```python
from build123d import *

# Parameters (mm, degrees)
SKETCH1_R           = 1.6
BOSS_EXTRUDE1_DEPTH = 3.175
SKETCH2_R           = 1.6
SKETCH2_R_2         = 7.5
CUT_EXTRUDE1_DEPTH  = 4.175


with BuildPart() as part:
    # Sketch1 → Boss-Extrude1 (new body)
    with BuildSketch(Plane.XY):
        with BuildLine():
            Line((31.086717458, 32.79124845), (24.539210672, 37.049362302))
            ThreePointArc((24.539210672, 37.049362302), (22.268882249, 37.695107847), (20.029743315, 36.948358029))
            Line((20.029743315, 36.948358029), (13.602836128, 32.346493758))
            ThreePointArc((13.602836128, 32.346493758), (12.968237383, 31.781029757), (12.467444066, 31.094246563))
            Line((12.467444066, 31.094246563), (1.349560594, 11.837507517))
            ThreePointArc((1.349560594, 11.837507517), (0.995156132, 11.028730142), (0.826837821, 10.16190126))
            Line((0.826837821, 10.16190126), (0.217529035, 2.673448792))
            ThreePointArc((0.217529035, 2.673448792), (0.712425098, 0.398045931), (2.390731369, -1.216162343))
            Line((2.390731369, -1.216162343), (9.39530455, -4.779380795))
            ThreePointArc((9.39530455, -4.779380795), (10.276421795, -5.10394936), (11.208926603, -5.214163404))
            Line((11.208926603, -5.214163404), (33.291073397, -5.214163404))
            ThreePointArc((33.291073397, -5.214163404), (34.223578205, -5.10394936), (35.10469545, -4.779380795))
            Line((35.10469545, -4.779380795), (42.181392008, -1.179473262))
            ThreePointArc((42.181392008, -1.179473262), (43.83187157, 0.385744129), (44.362149812, 2.597710054))
            Line((44.362149812, 2.597710054), (43.941412908, 10.526262814))
            ThreePointArc((43.941412908, 10.526262814), (43.781938908, 11.451617014), (43.411134666, 12.314296889))
            Line((43.411134666, 12.314296889), (32.370061269, 31.437996983))
            ThreePointArc((32.370061269, 31.437996983), (31.808360702, 32.190462814), (31.086717458, 32.79124845))
        make_face()
        with Locations((13.589745962, 17.846043489)):
            Circle(SKETCH1_R, mode=Mode.SUBTRACT)
        with Locations((9.526279442, 5.5)):
            Circle(SKETCH1_R, mode=Mode.SUBTRACT)
        with Locations((34.973720558, 5.5)):
            Circle(SKETCH1_R, mode=Mode.SUBTRACT)
        with Locations((30.910254038, 17.846043489)):
            Circle(SKETCH1_R, mode=Mode.SUBTRACT)
        with Locations((22.25, 27.538130468)):
            Circle(SKETCH1_R, mode=Mode.SUBTRACT)
        with Locations((22.25, 2.846043489)):
            Circle(SKETCH1_R, mode=Mode.SUBTRACT)
        with BuildLine():
            Line((42.370834875, 9.312177826), (35.370834875, -2.812177826))
            ThreePointArc((35.370834875, -2.812177826), (34.687822174, -2.995190528), (34.504809472, -2.312177826))
            Line((34.504809472, -2.312177826), (41.504809472, 9.812177826))
            ThreePointArc((41.504809472, 9.812177826), (42.187822174, 9.995190528), (42.370834875, 9.312177826))
        make_face(mode=Mode.SUBTRACT)
        with BuildLine():
            Line((10.01754221, -2.349929674), (3.01754221, 9.774425979))
            ThreePointArc((3.01754221, 9.774425979), (2.334529508, 9.957438681), (2.151516806, 9.274425979))
            Line((2.151516806, 9.274425979), (9.151516806, -2.849929674))
            ThreePointArc((9.151516806, -2.849929674), (9.834529508, -3.032942376), (10.01754221, -2.349929674))
        make_face(mode=Mode.SUBTRACT)
        with BuildLine():
            Line((15.358452868, 31.038130468), (29.358452868, 31.038130468))
            ThreePointArc((29.358452868, 31.038130468), (29.858452868, 31.538130468), (29.358452868, 32.038130468))
            Line((29.358452868, 32.038130468), (15.358452868, 32.038130468))
            ThreePointArc((15.358452868, 32.038130468), (14.858452868, 31.538130468), (15.358452868, 31.038130468))
        make_face(mode=Mode.SUBTRACT)
    extrude(amount=BOSS_EXTRUDE1_DEPTH)

    # Sketch2 → Cut-Extrude1 (cut, through all)
    with BuildSketch(Plane.XY.offset(3.175)):
        with Locations((41.761034996, 1.563830145)):
            Circle(SKETCH2_R)
        with Locations((2.789891826, 1.563830145)):
            Circle(SKETCH2_R)
        with Locations((22.275463411, 12.813830145)):
            Circle(SKETCH2_R_2)
        with Locations((22.275463411, 35.313830145)):
            Circle(SKETCH2_R)
    extrude(amount=-CUT_EXTRUDE1_DEPTH, mode=Mode.SUBTRACT)


solid = part.part
```
Geometry check sheet. Reference: the model listing, model coordinates, mm. A direction names the side the tool comes from. Coordinates: 2 decimals unless noted, no trailing zeros. Order: outer loops, then holes, each group sorted by start corner. A loop starts at its lowest first (then second) coordinate and runs counter-clockwise, first axis right, second up. Notation, with made-up numbers: (-29, -33.5) - (-24, -33.5) arc R20 ccw to (-24, -14.5) - close; hole circle Ø10 at (81, 64). An arc over 180 degrees is marked (long way). Use one line per item in the form item = value.
1. Draft check along X on faces 3 (the face through (10.26, -5.1, 1.57)), 4 (the face through (42.18, 10, 1.57)), 5 (the face through (43.786, 11.439, 1.565)). Enter one of: pulls with the +X half, pulls with the -X half, needs draft (parallel to the pull), parting line crosses it, or undercut.
Here are the results:
face_3 = pulls with the -X half
face_4 = undercut
face_5 = pulls with the +X half
2. Section check B-B (y = 14). Record the boundary of the cut face in (x, z) (3 decimals).
Here are the results:
outline = (2.598, 0) - (14.87, 0) - (14.87, 3.175) - (2.598, 3.175) - close; (29.681, 0) - (42.438, 0) - (42.438, 3.175) - (29.681, 3.175) - close
3. Section check D-D (x = 38). Record the boundary of the cut face in (y, z) (3 decimals), then the cut area to 3 significant figures.
Here are the results:
outline = (-3.307, 0) - (1.742, 0) - (1.742, 3.175) - (-3.307, 3.175) - close; (3.742, 0) - (21.687, 0) - (21.687, 3.175) - (3.742, 3.175) - close
area = 73.0 mm²
4. Section check C-C (x = 23). Record the boundary of the cut face in (y, z) (3 decimals), then the cut area to 3 significant figures.
Here are the results:
outline = (-5.214, 0) - (1.433, 0) - (1.433, 3.175) - (-5.214, 3.175) - close; (4.259, 0) - (5.349, 0) - (5.349, 3.175) - (4.259, 3.175) - close; (20.279, 0) - (26.125, 0) - (26.125, 3.175) - (20.279, 3.175) - close; (28.951, 0) - (31.038, 0) - (31.038, 3.175) - (28.951, 3.175) - close; (32.038, 0) - (33.887, 0) - (33.887, 3.175) - (32.038, 3.175) - close; (36.74, 0) - (37.644, 0) - (37.644, 3.175) - (36.74, 3.175) - close
area = 58.5 mm²
5. Scan lines: line 1 (Y direction, x = 22.25, z = 0.9); line 2 (Y direction, x = 15.5, z = 0.25); line 3 (X direction, y = -2, z = 1). Record each from-to range of solid material in increasing order.
Here are the results:
line_1 = -5.21 to 1.25, 4.45 to 5.31, 20.31 to 25.94, 29.14 to 31.04, 32.04 to 33.71, 36.91 to 37.69
line_2 = -5.21 to 9.6, 16.03 to 31.04, 32.04 to 33.7
line_3 = 3.93 to 8.66, 9.82 to 34.69, 35.84 to 40.57
6. Access from +Z, -Z, +X, -X, +Y, -Y to the whole of each face (thin tool, end or side, straight path). Record for faces 1 (the face through (14.86, 31.55, 1.57)), 2 (the face through (38.6, -3, 1.6)).
Here are the results:
face_1 = +Z, -Z
face_2 = +Z, -Z, +X, -Y
7. Section check A-A (x = 16.5). Record the boundary of the cut face in (y, z) (3 decimals).
Here are the results:
outline = (-5.214, 0) - (8.029, 0) - (8.029, 3.175) - (-5.214, 3.175) - close; (17.599, 0) - (31.038, 0) - (31.038, 3.175) - (17.599, 3.175) - close; (32.038, 0) - (34.421, 0) - (34.421, 3.175) - (32.038, 3.175) - close
